Part model, mm, in its own coordinate system. A direction names the side the tool comes from. Give positions to 0.01 mm unless a question says otherwise; leave off trailing zeros. Write each loop counter-clockwise with the first axis right and the second up, starting at its lowest first coordinate (ties: lowest second). Pieces come first, ordered by that corner, then holes.
from build123d import *

# Parameters (mm, degrees)
F0_R     = 20.5
F1_DEPTH = 20
F2_SIZE2 = 1
F2_SIZE  = 5
F3_T     = -2.5


with BuildPart() as f1:
    # F0 (on Top) → F1 (new body)
    with BuildSketch(Plane.XY):
        Circle(F0_R)
    extrude(amount=F1_DEPTH)

    # F2
    f2_edges = [f1.edges().sort_by_distance(p)[0] for p in [
        (-20.5, 0, 0),
    ]]
    chamfer(f2_edges, length=F2_SIZE, length2=F2_SIZE2)

    # F3
    f3_openings = [f1.faces().sort_by_distance(p)[0] for p in [
        (0, 0, 20),
    ]]
    offset(amount=F3_T, openings=f3_openings)


solid = f1.part
1) Saw through at C-C (z = 14.75). Write the cut outline in (x, y), and give its area (3 significant figures).
Check result:
outline: circle Ø41 at (0, 0); hole circle Ø36 at (0, 0)
area: 302 mm2
2) Mould opens along X. For faces 3 (the flat face through (1.4, -18.1, 20)), 4 (the conical face through (-15.5, -11.9, 0.2)), 5 (the flat face through (0, 0, 2.5)) say: +X half, -X half, draft (parallel to the pull), parting line (faces both ways), or undercut.
Check result:
face 3: draft
face 4: parting line
face 5: undercut
3) 3-axis set-ups, long thin cutter, end or side, ignore diameter. For faces 1 (the cylindrical face through (-2.343, 17.847, 12.521)), 2 (the flat face through (0, 0, 0)): which of +Z, -Z, +X, -X, +Y, -Y reach the whole face in a straight line?
Check result:
face 1: +Z
face 2: -Z, +X, -X, +Y, -Y
4) Flat gauge pins, fed straight in: P1, Ø12, axis at x = 11, z = 12, coming from the -Y side; P2, Ø6, axis at y = -4, z = 16, coming from the -X side; P3, Ø1.5, axis at x = -6.5, z = 7, coming from the +Y side. Where does each tip first touch, or does it go through?
Check result:
P1: stops at y = -19.88
P2: stops at x = -20.48
P3: stops at y = 19.68
5) Drill centre lines: L1, parallel to Y at x = 0, z = 12.5; L2, parallel to Z at x = 0, y = -16; L3, parallel to X at y = -0.5, z = 9. Where is each one in solid material? Low to high.
Check result:
L1: y = -20.5 to -18, 18 to 20.5
L2: z = 0 to 2.5
L3: x = -20.49 to -17.99, 17.99 to 20.49
6) Saw through at D-D (z = 4.5). Write the cut outline in (x, y), and give its area (3 significant figures).
Check result:
outline: circle Ø40.8 at (0, 0); hole circle Ø35.7 at (0, 0)
area: 306 mm2
7) Saw through at A-A (y = 0). Write the cut outline in (x, z).
Check result:
outline: (-20.5, 5) - (-19.5, 0) - (19.5, 0) - (20.5, 5) - (20.5, 20) - (18, 20) - (18, 5.25) - (17.45, 2.5) - (-17.45, 2.5) - (-18, 5.25) - (-18, 20) - (-20.5, 20) - close
